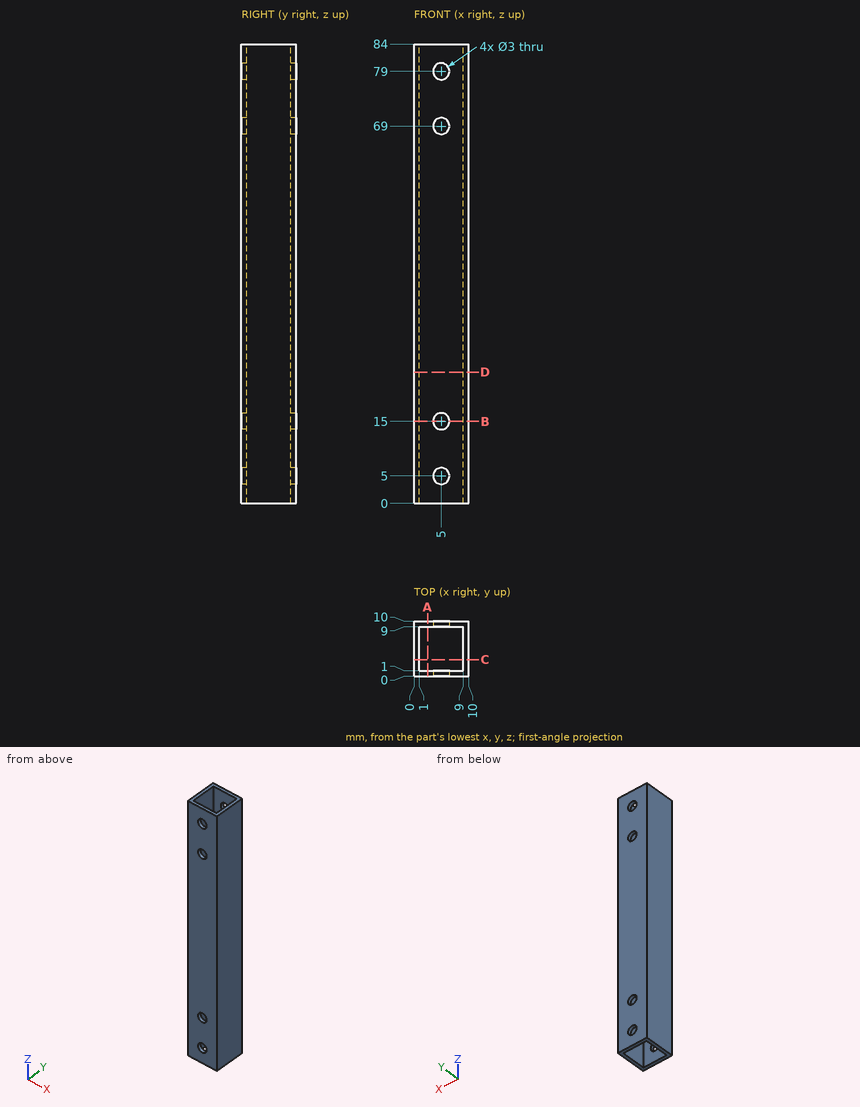
Source: three-view drawing plus pictorial views. Frame: mm from the lowest corner of the part. Round coordinates to 2 decimals unless told otherwise and drop trailing zeros. Loops run counter-clockwise (first coordinate to the right, second up) from the corner with the lowest first, then second, coordinate; pieces in that order, holes last.
Q1. Section A-A on x = 2.5. Return loops of the section in (y, z).
Q2. Material intervals for L1, parallel to Z at x = 5, y = 9.6; L2, parallel to Y at x = 4.25, z = 59.5, sorted ascending.
Q3. Section D-D on z = 24. Return loops of the section in (x, y).
Q4. Pin query (flat end, axial travel): P1, Ø2.5, axis at x = 5, z = 69, coming from the -Y side. Return the tip coordinate at first contact, or that it passes through.
Q5. Section B-B on z = 15. Return loops of the section in (x, y), plus the area to 3 significant figures.
Evaluation:
1. outline: (0, 0) - (1, 0) - (1, 84) - (0, 84) - close; (9, 0) - (10, 0) - (10, 84) - (9, 84) - close
2. L1: z = 0 to 3.5, 6.5 to 13.5, 16.5 to 67.5, 70.5 to 77.5, 80.5 to 84
2. L2: y = 0 to 1, 9 to 10
3. outline: (0, 0) - (10, 0) - (10, 10) - (0, 10) - close; hole (1, 1) - (9, 1) - (9, 9) - (1, 9) - close
4. P1: passes through
5. outline: (0, 0) - (3.5, 0) - (3.5, 1) - (1, 1) - (1, 9) - (3.5, 9) - (3.5, 10) - (0, 10) - close; (6.5, 0) - (10, 0) - (10, 10) - (6.5, 10) - (6.5, 9) - (9, 9) - (9, 1) - (6.5, 1) - close
5. area: 30.0 mm2
